Part model, mm, in its own coordinate system. A direction names the side the tool comes from. Round coordinates to 2 decimals unless told otherwise and drop trailing zeros. Loops run counter-clockwise (first coordinate to the right, second up) from the corner with the lowest first, then second, coordinate; pieces in that order, holes last.
1) Drop flat-ended pins along their axis: P1, Ø1.2, axis at x = 0, y = 6, coming from the -Z side; P2, Ø10, axis at y = -9.5, z = 34.5, coming from the -X side; P3, Ø7.5, axis at x = 0, y = 0, coming from the +Z side; P4, Ø10, axis at x = 4, z = 46, coming from the +Y side. Give the stop position or say it passes through.
2) Probe line 1 (Z direction, x = -3.25, y = -9); line 2 (Y direction, x = -7.5, z = 5.75); line 3 (X direction, y = 0.75, z = 14.5). List the from-to ranges inside material, lowest first.
3) Band-saw the part on A-A, the plane x = -7.5. Write the cut outline in (y, z), then the cut area to 3 significant figures.
4) Band-saw the part on B-B, the plane y = -8.5. Write the cut outline in (x, z), then the cut area to 3 significant figures.
5) Mould opens along X. For faces 1 (the cylindrical face through (-11.99, -0.53, 3.45)), 2 (the cylindrical face through (8.25, 0.03, 3.45)), 3 (the flat face through (5, -5, 0)) say: +X half, -X half, draft (parallel to the pull), parting line (faces both ways), or undercut.
6) 3-axis set-ups, long thin cutter, end or side, ignore diameter. For faces 4 (the flat face through (2, 3, 1)), 5 (the flat face through (-5, -5, 7)), 6 (the flat face through (-3, -3, 57)): which of +Z, -Z, +X, -X, +Y, -Y reach the whole face in a straight line?
7) Band-saw the part on C-C, the plane y = 0. State how many separate pieces and enclosed holes the cut face has, then the cut area to 3 significant figures.
Autodesk Inventor part; units mm, degrees
ref_plane "YZ Plane" through (0, 0, 0) normal (1, 0, 0) x (0, 1, 0)
ref_plane "XY Plane" through (0, 0, 0) normal (0, 0, 1) x (1, 0, 0)
sketch "Sketch1" plane through (0, 0, 0) normal (0, 0, 1) x (1, 0, 0)
  line L0 (0, 0) -> (0, 7.5)
  circle A0 centre (0, 7.5) radius 1.5
  circle A1 centre (-5.3033, 5.3033) radius 1.5
  circle A2 centre (-7.5, 0) radius 1.5
  circle A3 centre (-5.3033, -5.3033) radius 1.5
  circle A4 centre (0, -7.5) radius 1.5
  circle A5 centre (5.3033, -5.3033) radius 1.5
  circle A6 centre (7.5, 0) radius 1.5
  circle A7 centre (5.3033, 5.3033) radius 1.5
  circle A8 centre (0, 0) radius 12
  dimension "d0" = 7.5
  dimension "d1" = 3
  dimension "d4" = 360
  dimension "d6" = 24
extrude "Extrusion1" add sketch "Sketch1" along normal blind 7 contours A1 | A3 | A5 | A7 | A8
sketch "Sketch2" plane through (0, 0, 0) normal (0, 0, -1) x (-1, 0, 0)
  circle A0 centre (0, 0) radius 6.5
  dimension "d9" = 13
extrude "Extrusion2" cut sketch "Sketch2" against normal blind 1
sketch "Sketch3" plane through (0, 0, 7) normal (0, 0, 1) x (1, 0, 0)
  circle A0 centre (0, 0) radius 6.5
  dimension "d12" = 13
extrude "Extrusion3" add sketch "Sketch3" along normal blind 50
sketch "Sketch5" plane through (0, 0, 57) normal (0, 0, 1) x (1, 0, 0)
  circle A0 centre (0, 0) radius 3.25
  dimension "d25" = 6.5
extrude "Extrusion5" cut sketch "Sketch5" against normal up to surface (56 mm away)
ref_plane "Work Plane1" through (0, 12, 0) normal (0, 1, 0) x (-1, 0, 0)
sketch "Sketch8" plane through (0, 0, 7) normal (0, 0, 1) x (1, 0, 0)
  circle A0 centre (0, 0) radius 3
  dimension "d44" = 6
extrude "Extrusion8" cut sketch "Sketch8" against normal through all
sketch "Sketch9" plane through (0, 0, 0) normal (1, 0, 0) x (0, 1, 0)
  line L0 (6.5, 7) -> (6.5, 57)
  line L1 (6.5, 7) -> (6.5, 57)
  line L2 (6.4167, 7) -> (9, 7)
  line L3 (9, 7) -> (4, 7)
  line L4 (4, 7) -> (4, 14)
  line L5 (4, 14) -> (9, 14)
  line L6 (9, 14) -> (9, 7)
  line L7 (0, -11.4) -> (0, 68.4)
  point P0 (0, 0)
  dimension "d61" = 5
  dimension "d62" = 7
coil "Coil2" sketch "Sketch9" operation cut axis through (0, 0, 7) along (0, 0, 1) pitch 25 turns 2 hand right taper 1
sketch "Boceto13" plane through (0, 0, 0) normal (0, 0, -1) x (-1, 0, 0)
  arc A0 (-6.4167, 1.0375) -> (-6.4167, -1.0375) centre (-7.5, 0) ccw
  circle A1 centre (-7.5, 0) radius 1.5
  arc A2 (-1.0375, -6.4167) -> (1.0375, -6.4167) centre (0, -7.5) ccw
  circle A3 centre (0, -7.5) radius 1.5
  arc A4 (1.0375, 6.4167) -> (-1.0375, 6.4167) centre (0, 7.5) ccw
  circle A5 centre (0, 7.5) radius 1.5
  arc A6 (6.4167, -1.0375) -> (6.4167, 1.0375) centre (7.5, 0) ccw
  circle A7 centre (7.5, 0) radius 1.5
  point P0 (0, 0)
extrude "Extrusión9" add sketch "Boceto13" against normal blind 7
sketch "Boceto14" plane through (0, 0, 1) normal (0, 0, -1) x (-1, 0, 0)
  circle A0 centre (0, 0) radius 6.5
extrude "Extrusión10" cut sketch "Boceto14" along normal blind 2
sketch "Boceto15" plane through (0, 0, 0) normal (0, 0, -1) x (-1, 0, 0)
  line L0 (0, 0) -> (-7.5, 0)
  line L1 (0, 0) -> (7.5, 0)
  line L2 (0, 0) -> (0, 6)
  line L3 (0, 0) -> (0, -6)
  circle A0 centre (0, 6) radius 0.75
  circle A1 centre (-7.5, 0) radius 0.75
  circle A2 centre (0, -6) radius 0.75
  circle A3 centre (7.5, 0) radius 0.75
  dimension "d76" = 7.5
  dimension "d77" = 7.5
  dimension "d78" = 6
  dimension "d79" = 6
  dimension "d80" = 1.5
  dimension "d81" = 1.5
  dimension "d82" = 1.5
  dimension "d83" = 1.5
extrude "Extrusión11" cut sketch "Boceto15" against normal blind 7
properties part number "ScrewActuatorGripper"
Reported:
1. P1: stops at z = 7
1. P2: stops at x = -4.69
1. P3: stops at z = 57
1. P4: stops at y = 6.5
2. line 1: z = 0 to 7
2. line 2: y = -9.37 to -0.75, 0.75 to 9.37
2. line 3: x = -4.03 to -3.16, 3.16 to 6.46
3. outline: (-9.37, 0) - (-0.75, 0) - (-0.75, 7) - (-9.37, 7) - close; (0.75, 0) - (9.37, 0) - (9.37, 7) - (0.75, 7) - close
3. area: 121 mm2
4. outline: (-8.47, 0) - (8.47, 0) - (8.47, 7) - (-8.47, 7) - close
4. area: 119 mm2
5. face 1: parting line
5. face 2: undercut
5. face 3: draft
6. face 4: -Z
6. face 5: +Z
6. face 6: +Z, +X, -X, +Y, -Y
7. separate pieces: 4
7. enclosed holes: 0
7. area: 364 mm2
